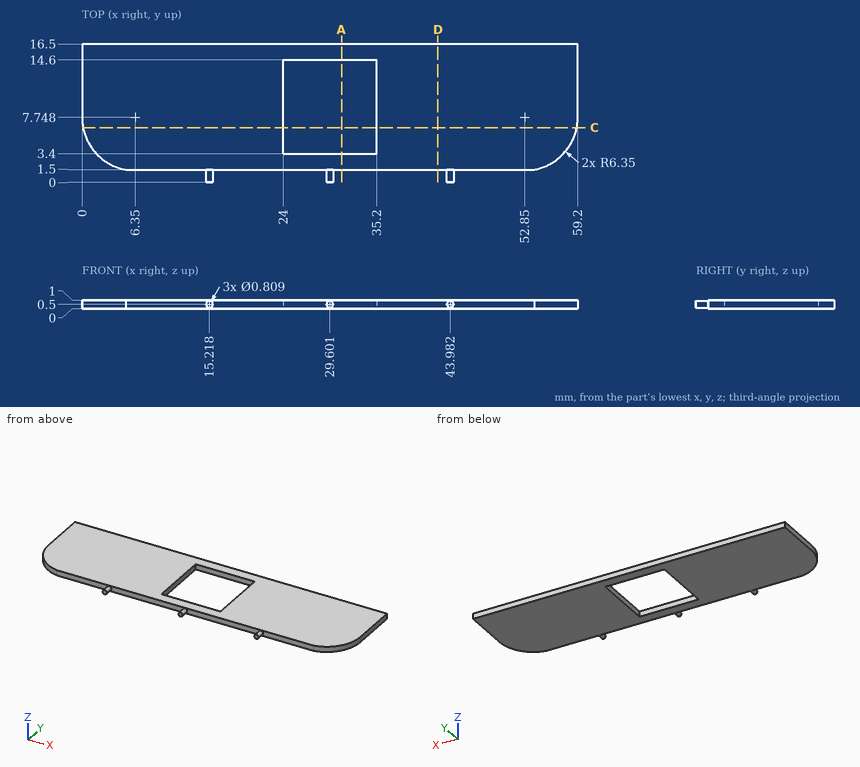
Can you work these out from the drawing? Everything is in mm from the part's minimum corner. Round coordinates to 2 decimals unless told otherwise and drop trailing zeros. Order: outer loops, then holes, each group sorted by start corner. A loop starts at its lowest first (then second) coordinate and runs counter-clockwise, first axis right, second up.
(1) If we section it at A-A (x = 31): Please give me the cut outline in (y, z).
Results are:
outline: (1.5, 0) - (3.4, 0) - (3.4, 1) - (1.5, 1) - close; (14.6, 0) - (16.5, 0) - (16.5, 1) - (14.6, 1) - close
(2) If we section it at C-C (y = 6.5): Please give me the cut outline in (x, z).
Results are:
outline: (0.12, 0) - (24, 0) - (24, 1) - (0.12, 1) - close; (35.2, 0) - (59.08, 0) - (59.08, 1) - (35.2, 1) - close
(3) If I drill on L1, parallel to Y at x = 27, z = 0.1; L2, parallel to X at y = 13.5, z = 0.3; L3, parallel to Y at x = 18.5, z = 0.75, over which ranges is the centre line in solid material (lowest first)?
Results are:
L1: y = 1.5 to 3.4, 14.6 to 16.5
L2: x = 0 to 24, 35.2 to 59.2
L3: y = 1.5 to 16.5
(4) I'm going to push a flat-ended pin straight in: pin 1 (5 mm diameter, centred on x = 30, y = 7.5, fed in from +Z). Where does the tip first touch, or does it pass through?
Results are:
pin 1: passes through
(5) If we section it at D-D (x = 42.5): Please give me the cut outline in (y, z), plus the area to 3 significant figures.
Results are:
outline: (1.5, 0) - (16.5, 0) - (16.5, 1) - (1.5, 1) - close
area: 15.0 mm2
